from build123d import *

# Parameters (mm, degrees)
F1_DEPTH = 2


with BuildPart() as f1:
    # F0 (on Front) → F1 (new body)
    with BuildSketch(Plane.XZ):
        with BuildLine():
            Line((-12.5, -15), (12.5, -15))
            Line((12.5, -15), (12.5, 15))
            Line((12.5, 15), (19.188319, 43.970291))
            Line((19.188319, 43.970291), (21.337286, 49.042992))
            Line((21.337286, 49.042992), (19.039087, 47.647727))
            Line((19.039087, 47.647727), (20.801328, 52.496947))
            Line((20.801328, 52.496947), (18.424573, 50.489065))
            Line((18.424573, 50.489065), (19.908065, 55.355389))
            Line((19.908065, 55.355389), (17.226272, 53.535521))
            Line((17.226272, 53.535521), (18.002436, 58.392484))
            Line((18.002436, 58.392484), (15.501298, 56.366656))
            Line((15.501298, 56.366656), (15.501298, 60.886702))
            Line((15.501298, 60.886702), (13.357465, 58.815028))
            Line((13.357465, 58.815028), (13.357465, 62.56105))
            Line((13.357465, 62.56105), (10.796777, 60.886702))
            Line((10.796777, 60.886702), (10.796777, 63.871168))
            Line((10.796777, 63.871168), (8.295841, 62.314177))
            Line((8.295841, 62.314177), (7.938334, 65.47904))
            Line((7.938334, 65.47904), (5.947843, 63.244458))
            Line((5.947843, 63.244458), (4.901238, 66.372305))
            Line((4.901238, 66.372305), (3.031312, 63.935702))
            Line((3.031312, 63.935702), (1.420656, 66.934533))
            Line((1.420656, 66.934533), (0, 64.162636))
            ThreePointArc((0, 64.162636), (-0.284516, 64.159145), (-0.568948, 64.151423))
            Line((-0.568948, 64.151423), (-2.127863, 66.794239))
            Line((-2.127863, 66.794239), (-3.23478, 63.871239))
            Line((-3.23478, 63.871239), (-4.81896, 65.873601))
            Line((-4.81896, 65.873601), (-5.945412, 63.184827))
            Line((-5.945412, 63.184827), (-7.934967, 65.02378))
            Line((-7.934967, 65.02378), (-8.529011, 62.109493))
            Line((-8.529011, 62.109493), (-8.599, 61.766136))
            Line((-8.599, 61.766136), (-8.828576, 61.954888))
            Line((-8.828576, 61.954888), (-10.83852, 63.607417))
            Line((-10.83852, 63.607417), (-11.411858, 60.316091))
            Line((-11.411858, 60.316091), (-13.175525, 61.766136))
            Line((-13.175525, 61.766136), (-13.733419, 58.252333))
            Line((-13.733419, 58.252333), (-15.767695, 59.924867))
            Line((-15.767695, 59.924867), (-15.767695, 55.726026))
            Line((-15.767695, 55.726026), (-17.302681, 57.800312))
            Line((-17.302681, 57.800312), (-17.302681, 52.987379))
            Line((-17.302681, 52.987379), (-19.411793, 54.721442))
            Line((-19.411793, 54.721442), (-18.347704, 50.112366))
            Line((-18.347704, 50.112366), (-20.197676, 51.63337))
            Line((-20.197676, 51.63337), (-18.985868, 46.384456))
            Line((-18.985868, 46.384456), (-21.409483, 48.377095))
            Line((-21.409483, 48.377095), (-18.884217, 42.653084))
            Line((-18.884217, 42.653084), (-12.5, 15))
            Line((-12.5, 15), (-12.5, -15))
        make_face()
    extrude(amount=F1_DEPTH)


solid = f1.part
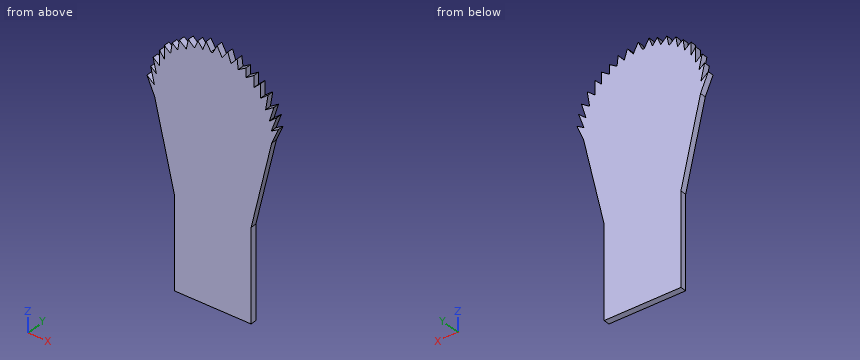
For this review, take the finished solid that the model builds, in its own axes (mm). Coordinates: 2 decimals unless noted, no trailing zeros. Order: outer loops, then holes, each group sorted by start corner. A loop starts at its lowest first (then second) coordinate and runs counter-clockwise, first axis right, second up. Notation, with made-up numbers: (-5.75, 74) - (34.25, 74) arc R16 ccw to (34.25, 85) - close; hole circle Ø5 at (-30.5, 84.25). An arc over 180 degrees is marked (long way). Use one line per item in the form item = value.
Q1. For probe 1 along X at (y, z) = (-0.55, 59); probe 2 along X at (y, z) = (-1.2, -0.5); probe 3 along Z at (x, y) = (2, -0.1), list the stretches that pass through material, from the lowest coordinate up. Write a range as from..to.
Checked values:
probe_1 = -15.77..-14.64, -13.61..13.36, 13.55..15.5
probe_2 = -12.5..12.5
probe_3 = -15..65.86
Q2. Consider section A-A (z = 8.5). Give the boundary of the cut face in (x, y).
Checked values:
outline = (-12.5, -2) - (12.5, -2) - (12.5, 0) - (-12.5, 0) - close
Q3. Consider section B-B (x = -4). Give the boundary of the cut face in (y, z).
Checked values:
outline = (-2, -15) - (0, -15) - (0, 64.84) - (-2, 64.84) - close
Q4. For P1, Ø0.6, axis at y = -1, z = 5.5, coming from the +X side; P2, Ø8, axis at x = -2.5, z = 57, coming from the +Y side; P3, Ø0.6, axis at y = -1.5, z = -6, coming from the -X side; P4, Ø0.6, axis at y = -0.5, z = 59, coming from the -X side, all flat-tipped, find the tip position at first contact; note any pin that passes through.
Checked values:
P1 = 12.5
P2 = 0
P3 = -12.5
P4 = -15.77
